Here's how the part is built. I have some questions about the finished solid (model axes, mm). Coordinates: 2 decimals unless noted, no trailing zeros. Loops run counter-clockwise (first coordinate to the right, second up) from the corner with the lowest first, then second, coordinate; pieces in that order, holes last. Notation, with made-up numbers: M 74.5,18.25 L 80.5,18.25 A16 ccw 80.5,37.25 Z; hole C -5.5,80.25 d1. An arc over 180 degrees is marked long. Use one line per item in the form item = value. Start each with the question number.
(1) Please list where these lines run through material, in increasing order: L1, parallel to X at y = 6.75, z = 0; L2, parallel to Z at x = 75.5, y = 3.5; L3, parallel to Z at x = 24, y = 6.
(2) Will these pins go through, and if not, where does the flat tip stop? P1, Ø6.5, axis at x = -11.25, z = -19.49, coming from the +Y side; P2, Ø5, axis at y = 7, z = -45, coming from the +X side.
(3) Imagine slicing it at C-C, the plane y = 8.5. State how many separate pieces and enclosed holes the cut face has, and give its area (3 significant figures).
(4) Imagine slicing it at B-B, the plane z = 0. Please give me the cut outline in (x, y), and give its area (3 significant figures).
(5) Imagine slicing it at A-A, the plane x = 11.25. Please give me the cut outline in (y, z).
(6) Imagine slicing it at D-D, the plane z = -42.5. Please give me the cut outline in (x, y).
```python
from build123d import *

# Parameters (mm, degrees)
BOSS_EXTRUDE1_DEPTH = 10
SKETCH2_R           = 15
CUT_EXTRUDE1_DEPTH  = 126.39936204
SKETCH2_3_R         = 15
SKETCH2_3_R_2       = 4
CUT_EXTRUDE2_DEPTH  = 5
CHAMFER1_SIZE       = 20


with BuildPart() as part:
    # Sketch1 → Boss-Extrude1 (new body)
    with BuildSketch(Plane(origin=(0, 0, 0), x_dir=(1, 0, 0), z_dir=(0, 1, 0))):
        Polygon((-80, 75), (-80, 15), (-60, 15), (-60, 75), (100, 75), (100, 55), (40, 55), (40, 35), (100, 35), (100, -75), (-100, -75), (-100, 75), align=None)
    extrude(amount=BOSS_EXTRUDE1_DEPTH)

    # Sketch2 → Cut-Extrude1 (cut, through all)
    with BuildSketch(Plane(origin=(0, 10, 0), x_dir=(1, 0, 0), z_dir=(0, 1, 0))):
        with Locations(Location((0, 0, 0), (0, 0, 270))):
            Circle(SKETCH2_R)
    extrude(amount=-CUT_EXTRUDE1_DEPTH, mode=Mode.SUBTRACT)

    # Sketch2_3 → Cut-Extrude2 (cut)
    with BuildSketch(Plane(origin=(0, 10, 0), x_dir=(1, 0, 0), z_dir=(0, 1, 0))):
        with Locations(Location((0, 0, 0), (0, 0, 270))):
            Circle(SKETCH2_3_R)
        with Locations(Location((22.5, 0, 0), (0, 0, 270))):
            Circle(SKETCH2_3_R_2)
        with Locations(Location((11.25, -19.485571585, 0), (0, 0, 270))):
            Circle(SKETCH2_3_R_2)
        with Locations(Location((-11.25, -19.485571585, 0), (0, 0, 270))):
            Circle(SKETCH2_3_R_2)
        with Locations(Location((-22.5, 0, 0), (0, 0, 270))):
            Circle(SKETCH2_3_R_2)
        with Locations(Location((-11.25, 19.485571585, 0), (0, 0, 270))):
            Circle(SKETCH2_3_R_2)
        with Locations(Location((11.25, 19.485571585, 0), (0, 0, 270))):
            Circle(SKETCH2_3_R_2)
        with BuildLine():
            ThreePointArc((-41.390750416, -53.951883934), (0, -68), (41.390750416, -53.951883934))
            ThreePointArc((41.390750416, -53.951883934), (42.86853083, -42.735103422), (31.651750318, -41.257323008))
            ThreePointArc((31.651750318, -41.257323008), (0, -52), (-31.651750318, -41.257323008))
            ThreePointArc((-31.651750318, -41.257323008), (-42.86853083, -42.735103422), (-41.390750416, -53.951883934))
        make_face()
    extrude(amount=-CUT_EXTRUDE2_DEPTH, mode=Mode.SUBTRACT)

    # Chamfer1
    chamfer1_edges = [part.edges().sort_by_distance(p)[0] for p in [
        (100, 5, 75),
    ]]
    chamfer(chamfer1_edges, length=CHAMFER1_SIZE)


solid = part.part
```
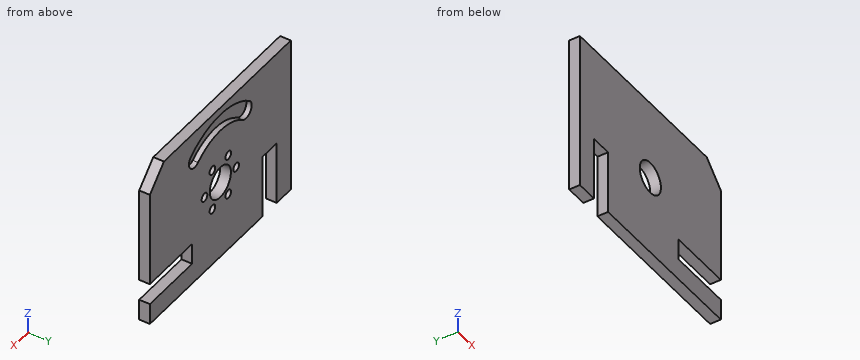
Answer:
q1.L1 = -100 to -26.5, -18.5 to -15, 15 to 18.5, 26.5 to 100
q1.L2 = -75 to -55, -35 to 75
q1.L3 = -75 to -3.71, 3.71 to 46.13, 63.62 to 75
q2.P1 = 5
q2.P2 = 40
q3.separate_pieces = 1
q3.enclosed_holes = 8
q3.area = 24,900 mm²
q4.outline = M -100,0 L -15,0 L -15,10 L -18.5,10 L -18.5,5 L -26.5,5 L -26.5,10 L -100,10 Z; M 15,0 L 100,0 L 100,10 L 26.5,10 L 26.5,5 L 18.5,5 L 18.5,10 L 15,10 Z
q4.area = 1,620 mm²
q5.outline = M 0,-75 L 10,-75 L 10,-23.49 L 5,-23.49 L 5,-15.49 L 10,-15.49 L 10,-9.92 L 0,-9.92 Z; M 0,9.92 L 10,9.92 L 10,15.49 L 5,15.49 L 5,23.49 L 10,23.49 L 10,50.77 L 5,50.77 L 5,67.06 L 10,67.06 L 10,75 L 0,75 Z
q6.outline = M -100,0 L -80,0 L -80,10 L -100,10 Z; M -60,0 L 40,0 L 40,10 L -60,10 Z
